Here's how the part is built. I have some questions about the finished solid (model axes, mm). Round coordinates to 2 decimals unless told otherwise and drop trailing zeros. Loops run counter-clockwise (first coordinate to the right, second up) from the corner with the lowest first, then second, coordinate; pieces in that order, holes last. Notation, with made-up numbers: M 14.5,-7 L 43.5,-7 A19 ccw 43.5,21 Z; hole C 59.5,74 d10. An arc over 180 degrees is marked long. Answer as a JSON object with one key per item and string values.
from build123d import *

# Parameters (mm, degrees)
SKETCH1_W           = 15.8
SKETCH1_H           = 15.8
BOSS_EXTRUDE1_DEPTH = 1.8
CUT_EXTRUDE1_REACH  = 13.316
SKETCH2_R           = 2.5
FILLET1_R           = 3.9
CHAMFER1_SIZE       = 1
CHAMFER1_SIZE2      = 1.732050808


with BuildPart() as part:
    # Sketch1 → Boss-Extrude1 (new body)
    with BuildSketch(Plane(origin=(0, 0, 0), x_dir=(1, 0, 0), z_dir=(0, 1, 0))):
        Rectangle(SKETCH1_W, SKETCH1_H)
    extrude(amount=BOSS_EXTRUDE1_DEPTH)

    # Sketch2 → Cut-Extrude1 (cut, up to next)
    with BuildSketch(Plane(origin=(0, 1.8, 0), x_dir=(1, 0, 0), z_dir=(0, 1, 0)), mode=Mode.PRIVATE) as cut_extrude1_sk1:
        with Locations(Location((-4, 4, 0), (0, 0, 270))):
            Circle(SKETCH2_R)
    cut_extrude1_tool1 = extrude(cut_extrude1_sk1.sketch, amount=-CUT_EXTRUDE1_REACH, mode=Mode.PRIVATE) & part.part
    # Sketch2 → Cut-Extrude1 (cut, up to next)
    with BuildSketch(Plane(origin=(0, 1.8, 0), x_dir=(1, 0, 0), z_dir=(0, 1, 0)), mode=Mode.PRIVATE) as cut_extrude1_sk2:
        with Locations(Location((4, 4, 0), (0, 0, 270))):
            Circle(SKETCH2_R)
    cut_extrude1_tool2 = extrude(cut_extrude1_sk2.sketch, amount=-CUT_EXTRUDE1_REACH, mode=Mode.PRIVATE) & part.part
    # Sketch2 → Cut-Extrude1 (cut, up to next)
    with BuildSketch(Plane(origin=(0, 1.8, 0), x_dir=(1, 0, 0), z_dir=(0, 1, 0)), mode=Mode.PRIVATE) as cut_extrude1_sk3:
        with Locations(Location((4, -4, 0), (0, 0, 270))):
            Circle(SKETCH2_R)
    cut_extrude1_tool3 = extrude(cut_extrude1_sk3.sketch, amount=-CUT_EXTRUDE1_REACH, mode=Mode.PRIVATE) & part.part
    # Sketch2 → Cut-Extrude1 (cut, up to next)
    with BuildSketch(Plane(origin=(0, 1.8, 0), x_dir=(1, 0, 0), z_dir=(0, 1, 0)), mode=Mode.PRIVATE) as cut_extrude1_sk4:
        with Locations(Location((-4, -4, 0), (0, 0, 270))):
            Circle(SKETCH2_R)
    cut_extrude1_tool4 = extrude(cut_extrude1_sk4.sketch, amount=-CUT_EXTRUDE1_REACH, mode=Mode.PRIVATE) & part.part
    add(cut_extrude1_tool1.solids().sort_by_distance((-4, 1.8, -4))[0], mode=Mode.SUBTRACT)
    add(cut_extrude1_tool2.solids().sort_by_distance((4, 1.8, -4))[0], mode=Mode.SUBTRACT)
    add(cut_extrude1_tool3.solids().sort_by_distance((4, 1.8, 4))[0], mode=Mode.SUBTRACT)
    add(cut_extrude1_tool4.solids().sort_by_distance((-4, 1.8, 4))[0], mode=Mode.SUBTRACT)

    # Fillet1
    fillet1_edges = [part.edges().sort_by_distance(p)[0] for p in [
        (-7.9, 0.9, -7.9),
        (7.9, 0.9, -7.9),
        (7.9, 0.9, 7.9),
        (-7.9, 0.9, 7.9),
    ]]
    fillet(fillet1_edges, radius=FILLET1_R)

    # Chamfer1
    chamfer1_edges = [part.edges().sort_by_distance(p)[0] for p in [
        (-4, 0, 1.5),
        (4, 0, 1.5),
        (4, 0, -6.5),
        (-4, 0, -6.5),
    ]]
    chamfer1_side = [part.faces().sort_by_distance(p)[0] for p in [
        (0, 0, 0),
    ]]
    chamfer(chamfer1_edges, length=CHAMFER1_SIZE, length2=CHAMFER1_SIZE2, reference=chamfer1_side[0])


solid = part.part
Item 1: I want a section at A-A, the plane y = 0.5. Please give me the cut outline in (x, z), then the cut area to 3 significant figures.
Resolved:
{"outline": "M -7.9,-4 A3.9 ccw -4,-7.9 L 4,-7.9 A3.9 ccw 7.9,-4 L 7.9,4 A3.9 ccw 4,7.9 L -4,7.9 A3.9 ccw -7.9,4 Z; hole C -4,-4 d6.42; hole C -4,4 d6.42; hole C 4,-4 d6.42; hole C 4,4 d6.42", "area": "107 mm²"}
Item 2: Please list where these lines run through material, in increasing order: probe 1 along X at (y, z) = (0.15, -2.5); probe 2 along Z at (x, y) = (-1.75, 1.35); probe 3 along X at (y, z) = (0.35, -2). Write a range as from..to.
Resolved:
{"probe 1": "-7.9..-7.07, -0.93..0.93, 7.07..7.9", "probe 2": "-7.9..-5.53, -2.47..2.47, 5.53..7.9", "probe 3": "-7.9..-6.62, -1.38..1.38, 6.62..7.9"}
Item 3: I want a section at B-B, the plane z = 3.5. State how many separate pieces and enclosed holes the cut face has, then the cut area to 3 significant figures.
Resolved:
{"separate pieces": "3", "enclosed holes": "0", "area": "7.28 mm²"}
Item 4: I'm going to push a flat-ended pin straight in: pin 1 Ø3 at (x, z) = (4, -4) entering from -Y. Where does the tip first touch, or does it pass through?
Resolved:
{"pin 1": "through"}
